For this review, take the finished solid that the model builds, in its own axes (mm). Coordinates: 2 decimals unless noted, no trailing zeros. Loops run counter-clockwise (first coordinate to the right, second up) from the corner with the lowest first, then second, coordinate; pieces in that order, holes last.
1. To check wall thickness, follow probe 1 along Y at (x, z) = (0, 4); probe 2 along X at (y, z) = (3, 7); probe 3 along X at (y, z) = (169, 1.75). State the ranges of each line that lie inside material, in increasing order.
2. Take a section at D-D, the plane y = -228. State the section outline as (x, z) points, then the cut area to 3 significant figures.
3. Take a section at A-A, the plane x = 0. State the section outline as (y, z) points.
4. Clearance check with flat-ended pins moving along their axes: P1, Ø4, axis at x = -9.5, z = 9, coming from the -Y side; P2, Ø6.5, axis at x = -1.5, z = 8.5, coming from the +Y side; P3, Ø4, axis at y = -8.5, z = 6.5, coming from the -X side. State where each tip first meets the part, or that it passes through.
5. Take a section at C-C, the plane y = 254. State the section outline as (x, z) points, then the cut area to 3 significant figures.
6. Take a section at B-B, the plane z = 2.25. Count the separate pieces of the cut face and the enclosed holes in it, then the cut area to 3 significant figures.
```python
from build123d import *

# Parameters (mm, degrees)
F1_DEPTH = 12.7


with BuildPart() as f1:
    # F0 (on Top) → F1 (new body)
    with BuildSketch(Plane.XY):
        with BuildLine():
            Line((166.6875, -333.375), (166.6875, -166.6875))
            Line((166.6875, -166.6875), (127, -166.6875))
            ThreePointArc((127, -166.6875), (0, -293.6875), (-127, -166.6875))
            Line((-127, -166.6875), (-166.6875, -166.6875))
            Line((-166.6875, -166.6875), (-166.6875, -333.375))
            Line((-166.6875, -333.375), (-19.05, -333.375))
            Line((-19.05, -333.375), (-19.05, -317.5))
            Line((-19.05, -317.5), (19.05, -317.5))
            Line((19.05, -317.5), (19.05, -333.375))
            Line((19.05, -333.375), (166.6875, -333.375))
        make_face()
        with BuildLine():
            Line((127, 166.6875), (166.6875, 166.6875))
            Line((166.6875, 166.6875), (166.6875, 333.375))
            Line((166.6875, 333.375), (19.05, 333.375))
            Line((19.05, 333.375), (19.05, 317.5))
            Line((19.05, 317.5), (-19.05, 317.5))
            Line((-19.05, 317.5), (-19.05, 333.375))
            Line((-19.05, 333.375), (-166.6875, 333.375))
            Line((-166.6875, 333.375), (-166.6875, 166.6875))
            Line((-166.6875, 166.6875), (-127, 166.6875))
            ThreePointArc((-127, 166.6875), (0, 293.6875), (127, 166.6875))
        make_face()
        with BuildLine():
            Line((127, -166.6875), (166.6875, -166.6875))
            Line((166.6875, -166.6875), (166.6875, -19.05))
            Line((166.6875, -19.05), (150.8125, -19.05))
            Line((150.8125, -19.05), (150.8125, 19.05))
            Line((150.8125, 19.05), (166.6875, 19.05))
            Line((166.6875, 19.05), (166.6875, 166.6875))
            Line((166.6875, 166.6875), (127, 166.6875))
            ThreePointArc((127, 166.6875), (0, 39.6875), (-127, 166.6875))
            Line((-127, 166.6875), (-166.6875, 166.6875))
            Line((-166.6875, 166.6875), (-166.6875, 19.05))
            Line((-166.6875, 19.05), (-150.8125, 19.05))
            Line((-150.8125, 19.05), (-150.8125, -19.05))
            Line((-150.8125, -19.05), (-166.6875, -19.05))
            Line((-166.6875, -19.05), (-166.6875, -166.6875))
            Line((-166.6875, -166.6875), (-127, -166.6875))
            ThreePointArc((-127, -166.6875), (0, -39.6875), (127, -166.6875))
        make_face()
    extrude(amount=F1_DEPTH)


solid = f1.part
```
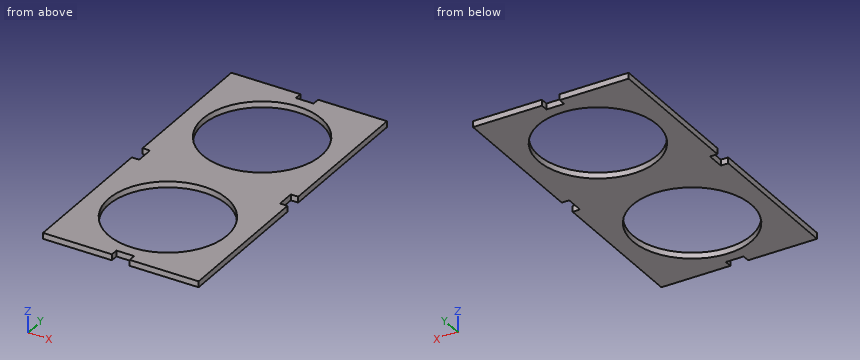
Results list:
1. probe 1: y = -317.5 to -293.69, -39.69 to 39.69, 293.69 to 317.5
1. probe 2: x = -150.81 to 150.81
1. probe 3: x = -166.69 to -126.98, 126.98 to 166.69
2. outline: (-166.69, 0) - (-111.22, 0) - (-111.22, 12.7) - (-166.69, 12.7) - close; (111.22, 0) - (166.69, 0) - (166.69, 12.7) - (111.22, 12.7) - close
2. area: 1,410 mm2
3. outline: (-317.5, 0) - (-293.69, 0) - (-293.69, 12.7) - (-317.5, 12.7) - close; (-39.69, 0) - (39.69, 0) - (39.69, 12.7) - (-39.69, 12.7) - close; (293.69, 0) - (317.5, 0) - (317.5, 12.7) - (293.69, 12.7) - close
4. P1: stops at y = -317.5
4. P2: stops at y = 317.5
4. P3: stops at x = -150.81
5. outline: (-166.69, 0) - (-92.23, 0) - (-92.23, 12.7) - (-166.69, 12.7) - close; (92.23, 0) - (166.69, 0) - (166.69, 12.7) - (92.23, 12.7) - close
5. area: 1,890 mm2
6. separate pieces: 1
6. enclosed holes: 2
6. area: 119,000 mm2
